Geometry check sheet. Reference: drawing and pictorial views, mm from the part's lowest x, y, z. Round coordinates to 2 decimals unless told otherwise and drop trailing zeros. Write each loop counter-clockwise with the first axis right and the second up, starting at its lowest first coordinate (ties: lowest second). Pieces come first, ordered by that corner, then holes.
Item 1: Release check for a two-part mould opening along X. For the marked faces 1, 2, 3 and 4 record: pulls with the +X half, pulls with the -X half, needs draft (parallel to the pull), parting line crosses it, or undercut.
Item 2: Section check A-A, the plane y = 3. Record the cut outline in (x, z).
Item 3: Depth check by flat-ended pin: pin 1 (2.5 mm diameter, centred on x = 3, y = 3, fed in from -Z). Enter the tip coordinate at first touch or a pass-through.
Item 4: Section check C-C, the plane z = 1.4. Record the cut outline in (x, y).
Item 5: Material ranges on line 1 along Y through (x, z) = (3, 4.3); line 2 along X through (y, z) = (3.5, 3.65) (1 decimal); line 3 along X through (y, z) = (3.75, 5.25) (1 decimal), recorded low to high.
Item 6: Section check B-B, the plane x = 3. Record the cut outline in (y, z).
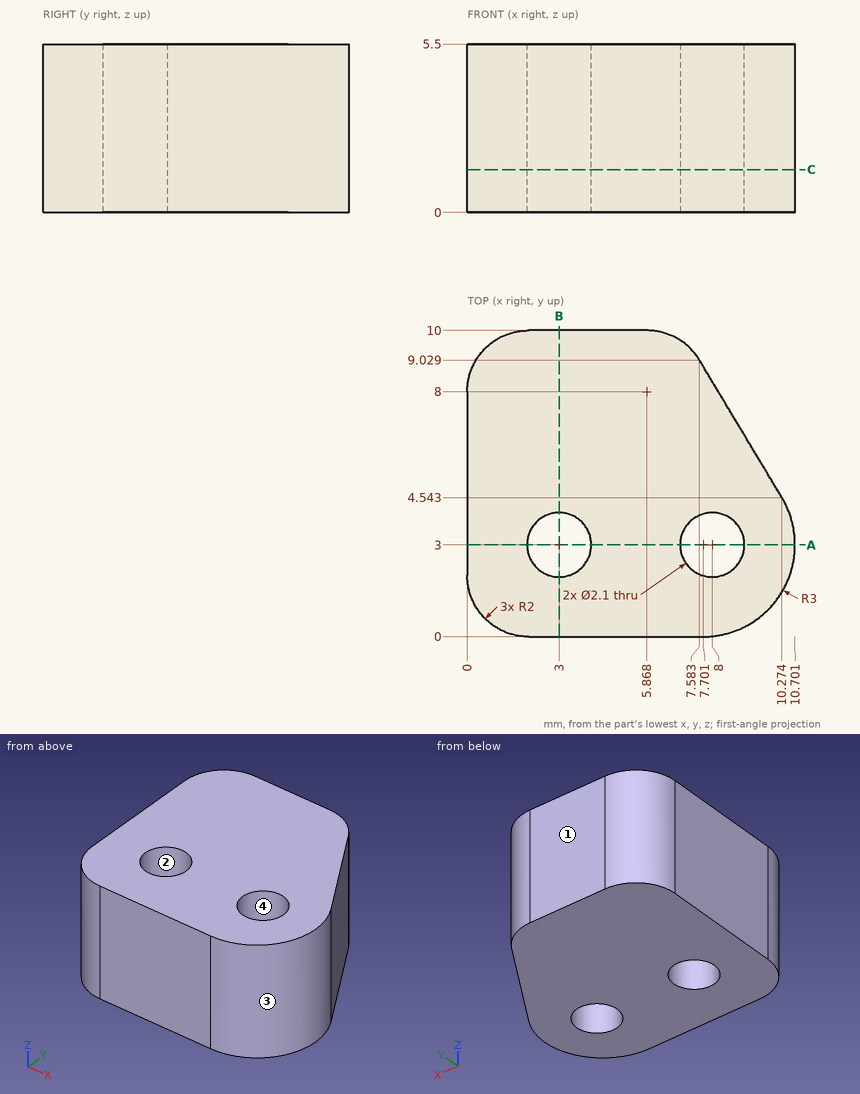
Values found:
1. face 1: needs draft
1. face 2: undercut
1. face 3: pulls with the +X half
1. face 4: undercut
2. outline: (0, 0) - (1.95, 0) - (1.95, 5.5) - (0, 5.5) - close; (4.05, 0) - (6.95, 0) - (6.95, 5.5) - (4.05, 5.5) - close; (9.05, 0) - (10.7, 0) - (10.7, 5.5) - (9.05, 5.5) - close
3. pin 1: stops at z = 0
4. outline: (0, 2) arc R2 ccw to (2, 0) - (7.7, 0) arc R3 ccw to (10.27, 4.54) - (7.58, 9.03) arc R2 ccw to (5.87, 10) - (2, 10) arc R2 ccw to (0, 8) - close; hole circle Ø2.1 at (3, 3); hole circle Ø2.1 at (8, 3)
5. line 1: y = 0 to 1.95, 4.05 to 10
5. line 2: x = 0 to 2.1, 3.9 to 7.1, 8.9 to 10.7
5. line 3: x = 0 to 2.3, 3.7 to 7.3, 8.7 to 10.6
6. outline: (0, 0) - (1.95, 0) - (1.95, 5.5) - (0, 5.5) - close; (4.05, 0) - (10, 0) - (10, 5.5) - (4.05, 5.5) - close
